The listing builds one solid part. Answer for the finished solid, in the listing's coordinates (mm). Face numbers are marked on the shaded views. A direction names the side the tool comes from. Round coordinates to 2 decimals unless told otherwise and drop trailing zeros. Order: outer loops, then holes, each group sorted by start corner. A loop starts at its lowest first (then second) coordinate and runs counter-clockwise, first axis right, second up. Notation, with made-up numbers: M 82.25,61 L 112.25,61 A20 ccw 112.25,95 Z; hole C 61,16.25 d3. An arc over 180 degrees is marked long. Write item = value, one per line. Start each with the question number.
(1) Straight lines are drawn through the part: probe 1 along X at (y, z) = (2.5, -12.5); probe 2 along X at (y, z) = (0, -14); probe 3 along Z at (x, y) = (-2.75, -3.5). For each, find the intervals that lie inside material, in ascending order. Write a range as from..to.
(2) A cutting plane is placed at D-D, the plane y = 3. Count the separate pieces of the cut face and the enclosed holes in it, and give its area (3 significant figures).
(3) For a pull along Z with two mould halves and no side action, classify the marked faces 1, 2 and 3 as released by +Z, released by -Z, zero draft, split by the parting line, or undercut.
(4) A cutting plane is placed at A-A, the plane z = -7.5. Determine the outline of the cut face in (x, y), and give its area (3 significant figures).
(5) A cutting plane is placed at B-B, the plane z = -12.5. Determine the outline of the cut face in (x, y).
(6) A cutting plane is placed at C-C, the plane x = 4. Determine the outline of the cut face in (y, z).
(7) This flat-tipped pin is pushed along its axis until it touches: pin 1 (3 mm diameter, centred on x = 0, y = 0, fed in from -Z). Where does it stop, or does it pass through?
(8) Which of the six approach directions +Z, -Z, +X, -X, +Y, -Y give full straight-line access (tool end or side, diameter ignored) to the marked faces 4 and 5?
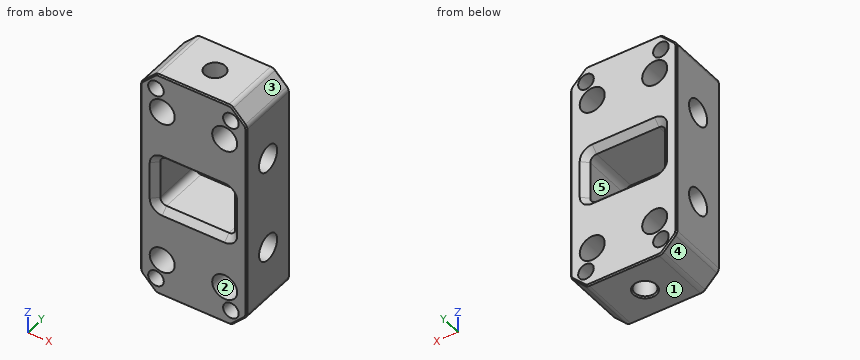
from build123d import *
from OCP.BRepFilletAPI import BRepFilletAPI_MakeChamfer

# Parameters (mm, degrees)
SKETCH_1_W          = 17
SKETCH_1_H          = 37
EXTRUDE_1_DEPTH     = 5
SKETCH_2_R          = 1.5
CUT_EXTRUDE_1_DEPTH = 26.617376915
SKETCH_3_R          = 1.6
CUT_EXTRUDE_3_DEPTH = 8
SKETCH_4_R          = 1
SKETCH_4_W          = 12
SKETCH_4_H          = 8
CUT_EXTRUDE_4_DEPTH = 23.682592444
CHAMFER_1_SIZE      = 2.5
SKETCH_6_R          = 2
CUT_EXTRUDE_5_DEPTH = 23.682592444
FILLET_1_R          = 1
HOLE_WIZARD_M3_1_D  = 2.5
CHAMFER_2_SIZE      = 0.2
CHAMFER_2_SIZE2     = 0.584574438
CHAMFER_3_SIZE      = 0.2
CHAMFER_4_SIZE      = 1
HOLE_WIZARD_M5_1_D  = 4.2


# Read off the part's stored shape, not the designer's step: M4 螺纹孔1
with BuildPart() as part:
    # 草图1 → 凸台-拉伸1 (new, symmetric)
    with BuildSketch(Plane(origin=(0, 0, 0), x_dir=(1, 0, 0), z_dir=(0, 1, 0))):
        Rectangle(SKETCH_1_W, SKETCH_1_H)
    extrude(amount=EXTRUDE_1_DEPTH, both=True)

    # 草图2 → 切除-拉伸1 (cut, through all)
    with BuildSketch(Plane(origin=(8.5, 0, 0), x_dir=(0, 0, -1), z_dir=(1, 0, 0))):
        with Locations((-7.5, 0)):
            Circle(SKETCH_2_R)
        with Locations((7.5, 0)):
            Circle(SKETCH_2_R)
    extrude(amount=-CUT_EXTRUDE_1_DEPTH, mode=Mode.SUBTRACT)

    # 草图3 → 切除-拉伸3 (cut)
    with BuildSketch(Plane(origin=(0, 0, -18.5), x_dir=(-1, 0, 0), z_dir=(0, 0, -1))):
        Circle(SKETCH_3_R)
    cut_extrude_3 = extrude(amount=-CUT_EXTRUDE_3_DEPTH, mode=Mode.SUBTRACT)

    # 草图4 → 切除-拉伸4 (cut, through all)
    with BuildSketch(Plane(origin=(0, 5, 0), x_dir=(1, 0, 0), z_dir=(0, 1, 0))):
        with Locations(Location((-6, -16, 0), (0, 0, 270))):
            Circle(SKETCH_4_R)
        with Locations(Location((6, -16, 0), (0, 0, 270))):
            Circle(SKETCH_4_R)
        with Locations(Location((6, 16, 0), (0, 0, 270))):
            Circle(SKETCH_4_R)
        with Locations(Location((-6, 16, 0), (0, 0, 270))):
            Circle(SKETCH_4_R)
        Rectangle(SKETCH_4_W, SKETCH_4_H)
    extrude(amount=-CUT_EXTRUDE_4_DEPTH, mode=Mode.SUBTRACT)

    # 镜向1: 切除-拉伸3 across plane
    add(cut_extrude_3.mirror(Plane.XY), mode=Mode.SUBTRACT)

    # 倒角1
    chamfer_1_edges = [part.edges().sort_by_distance(p)[0] for p in [
        (8.5, 0, 18.5),
        (-8.5, 0, 18.5),
        (-8.5, 0, -18.5),
        (8.5, 0, -18.5),
    ]]
    chamfer(chamfer_1_edges, length=CHAMFER_1_SIZE)

    # 草图6 → 切除-拉伸5 (cut, through all)
    with BuildSketch(Plane(origin=(0, 5, 0), x_dir=(1, 0, 0), z_dir=(0, 1, 0))):
        with Locations(Location((5, 12.5, 0), (0, 0, 270))):
            Circle(SKETCH_6_R)
        with Locations(Location((-5, 12.5, 0), (0, 0, 270))):
            Circle(SKETCH_6_R)
        with Locations(Location((5, -12.5, 0), (0, 0, 270))):
            Circle(SKETCH_6_R)
        with Locations(Location((-5, -12.5, 0), (0, 0, 270))):
            Circle(SKETCH_6_R)
    extrude(amount=-CUT_EXTRUDE_5_DEPTH, mode=Mode.SUBTRACT)

    # 圆角1
    fillet_1_edges = [part.edges().sort_by_distance(p)[0] for p in [
        (6, 0, -4),
        (6, 0, 4),
        (-6, 0, 4),
        (-6, 0, -4),
        (-8.5, 0, 16),
        (-8.5, 0, -16),
        (6, 0, -18.5),
        (-6, 0, -18.5),
        (8.5, 0, 16),
        (8.5, 0, -16),
        (-6, 0, 18.5),
        (6, 0, 18.5),
    ]]
    fillet(fillet_1_edges, radius=FILLET_1_R)

    # M4 螺纹孔1 outline → M4 螺纹孔1 (revolve, cut)
    with BuildSketch(Plane.XZ):
        Polygon((0, -9.508579979), (0, -10.5), (1.6, -10.5), (1.6, -18.5), (1.65, -18.5), (1.65, -10.5), align=None)
        Polygon((0, 10.5), (0, 9.508579979), (1.65, 10.5), (1.65, 18.5), (1.6, 18.5), (1.6, 10.5), align=None)
    revolve(axis=Axis((0, 0, 0), (0, 0, 1)), mode=Mode.SUBTRACT)

    # M3 螺纹孔1 (through all)
    with Locations(Plane(origin=(0, 5, 0), x_dir=(1, 0, 0), z_dir=(0, 1, 0))):
        with Locations((-6, -16), (6, -16), (6, 16), (-6, 16)):
            Hole(HOLE_WIZARD_M3_1_D / 2)

    # 倒角2: one chamfer whose edges measure the first distance from different faces: ONE call of the kernel's chamfer builder (chamfer() names one face for all edges)
    chamfer_2_edges_1 = [part.edges().sort_by_distance(p)[0] for p in [
        (-8.5, 5, 0),
        (0, 5, -18.5),
        (-7.25, 5, -17.25),
        (-7.25, 5, 17.25),
        (0, 5, 18.5),
        (7.25, 5, 17.25),
        (8.5, 5, 0),
        (7.25, 5, -17.25),
        (5.96846987, 5, 18.423879533),
        (-8.423879533, 5, -15.96846987),
        (-5.96846987, 5, -18.423879533),
        (5.96846987, 5, -18.423879533),
        (8.423879533, 5, -15.96846987),
        (8.423879533, 5, 15.96846987),
        (-5.96846987, 5, 18.423879533),
        (-8.423879533, 5, 15.96846987),
        (-1.65, 0, -18.5),
    ]]
    chamfer_2_edges_2 = [part.edges().sort_by_distance(p)[0] for p in [
        (-1.65, 0, -10.5),
    ]]
    chamfer_2_side_2 = [part.faces().sort_by_distance(p)[0] for p in [
        (-1.65, 0, -14.5),
    ]]
    chamfer_2 = BRepFilletAPI_MakeChamfer(part.part.solid().wrapped)
    for e in chamfer_2_edges_1:
        chamfer_2.Add(CHAMFER_2_SIZE, e.wrapped)
    for e in chamfer_2_edges_2:
        chamfer_2.Add(CHAMFER_2_SIZE, CHAMFER_2_SIZE2, e.wrapped, chamfer_2_side_2[0].wrapped)  # the first distance lies on this face
    add(Compound.cast(chamfer_2.Shape()), mode=Mode.REPLACE)

    # 倒角3
    chamfer_3_edges = [part.edges().sort_by_distance(p)[0] for p in [
        (-8.5, -5, 0),
        (-7.25, -5, 17.25),
        (-7.25, -5, -17.25),
        (0, -5, -18.5),
        (7.25, -5, -17.25),
        (8.5, -5, 0),
        (7.25, -5, 17.25),
        (0, -5, 18.5),
        (5.96846987, -5, 18.423879533),
        (-8.423879533, -5, -15.96846987),
        (-5.96846987, -5, -18.423879533),
        (5.96846987, -5, -18.423879533),
        (8.423879533, -5, -15.96846987),
        (8.423879533, -5, 15.96846987),
        (-5.96846987, -5, 18.423879533),
        (-8.423879533, -5, 15.96846987),
    ]]
    chamfer(chamfer_3_edges, length=CHAMFER_3_SIZE)

    # 倒角4
    chamfer_4_edges = [part.edges().sort_by_distance(p)[0] for p in [
        (6, 5, 0),
        (0, 5, 4),
        (-6, 5, 0),
        (0, 5, -4),
        (0, -5, 4),
        (6, -5, 0),
        (0, -5, -4),
        (-6, -5, 0),
        (-5.707106781, 5, 3.707106781),
        (-5.707106781, -5, 3.707106781),
        (-5.707106781, 5, -3.707106781),
        (-5.707106781, -5, -3.707106781),
        (5.707106781, 5, -3.707106781),
        (5.707106781, -5, -3.707106781),
        (5.707106781, 5, 3.707106781),
        (5.707106781, -5, 3.707106781),
    ]]
    chamfer(chamfer_4_edges, length=CHAMFER_4_SIZE)

    # M5 螺纹孔1 (through all)
    with Locations(Plane(origin=(8.5, 0, 0), x_dir=(0, 0, -1), z_dir=(1, 0, 0))):
        with Locations((-7.5, 0), (7.5, 0)):
            Hole(HOLE_WIZARD_M5_1_D / 2)


solid = part.part
Reported:
q1.probe_1 = -8.5..-7, -3..3, 7..8.5
q1.probe_2 = -8.5..-6.32, -3.68..-1.65, 1.65..3.68, 6.32..8.5
q1.probe_3 = -18.5..-4, 4..18.5
q2.separate_pieces = 1
q2.enclosed_holes = 9
q2.area = 451 mm²
q3.face_1 = released by -Z
q3.face_2 = undercut
q3.face_3 = released by +Z
q4.outline = M -8.5,-4.8 L -8.3,-5 L 8.3,-5 L 8.5,-4.8 L 8.5,-2.1 L -8.5,-2.1 Z; M -8.5,2.1 L 8.5,2.1 L 8.5,4.8 L 8.3,5 L -8.3,5 L -8.5,4.8 Z
q4.area = 98.5 mm²
q5.outline = M -8.5,-4.8 L -8.3,-5 L -7,-5 L -7,5 L -8.3,5 L -8.5,4.8 Z; M -3,-5 L 3,-5 L 3,5 L -3,5 Z; M 7,-5 L 8.3,-5 L 8.5,-4.8 L 8.5,4.8 L 8.3,5 L 7,5 Z; hole C 0,0 d3.3
q6.outline = M -5,-18.3 L -4.8,-18.5 L 4.8,-18.5 L 5,-18.3 L 5,-14.23 L -5,-14.23 Z; M -5,-10.77 L 5,-10.77 L 5,-5 L 4,-4 L -4,-4 L -5,-5 Z; M -5,5 L -4,4 L 4,4 L 5,5 L 5,10.77 L -5,10.77 Z; M -5,14.23 L 5,14.23 L 5,18.3 L 4.8,18.5 L -4.8,18.5 L -5,18.3 Z; hole C 0,-7.5 d4.2; hole C 0,7.5 d4.2
q7.pin_1 = -10.55
q8.face_4 = -Z, -X, +Y, -Y
q8.face_5 = +Y, -Y
